```python
from build123d import *

# Parameters (mm, degrees)
BOSS_EXTRUDE1_DEPTH = 29.337
SKETCH1_R           = 5.842
BOSS_EXTRUDE2_DEPTH = 1.27
BOSS_EXTRUDE3_DEPTH = 12.7


with BuildPart() as part:
    # Sketch 1 → Boss-Extrude1 (new, symmetric)
    with BuildSketch(Plane.XY):
        Polygon((7.3025, 0), (3.65125, 6.324150511), (-3.65125, 6.324150511), (-7.3025, 0), (-3.65125, -6.324150511), (3.65125, -6.324150511), align=None)
    extrude(amount=BOSS_EXTRUDE1_DEPTH, both=True)

    # Sketch1 → Boss-Extrude2 (add)
    with BuildSketch(Plane(origin=(0, 0, -29.337), x_dir=(-1, 0, 0), z_dir=(0, 0, -1))):
        with Locations(Location((0, 0, 0), (0, 0, 180))):
            Circle(SKETCH1_R)
    extrude(amount=BOSS_EXTRUDE2_DEPTH)

    # Sketch2 → Boss-Extrude3 (add)
    with BuildSketch(Plane(origin=(0, 0, -30.607), x_dir=(-1, 0, 0), z_dir=(0, 0, -1))):
        Polygon((3.729553625, -6.278290851), (7.301936182, 0.090742758), (3.572382557, 6.369033609), (-3.729553625, 6.278290851), (-7.301936182, -0.090742758), (-3.572382557, -6.369033609), align=None)
    extrude(amount=BOSS_EXTRUDE3_DEPTH)


solid = part.part
```
Input: part model. Units: mm. Frame: model coordinates. Give positions to 0.01 mm unless a question says otherwise; leave off trailing zeros. Order: outer loops, then holes, each group sorted by start corner. A loop starts at its lowest first (then second) coordinate and runs counter-clockwise, first axis right, second up. Notation, with made-up numbers: M 0.25,-23 L 41.25,-23 A14 cw 41.25,-8 Z; hole C 15,-37 d2. An arc over 180 degrees is marked long. One line per question, with ' | ' between items.
1) Contact query for flat-ended pins moving along their axis: P1, Ø6, axis at x = -2, z = 17, coming from the -Y side; P2, Ø2, axis at x = -3.5, z = -1, coming from the +Y side; P3, Ø1, axis at x = -4.5, z = -6, coming from the +Y side. Output: stop coordinate, or through.
Filled in:
P1: stops at y = -6.32 | P2: stops at y = 6.32 | P3: stops at y = 5.72
2) Draft query along Z for faces 1 (the face through (0, 0, -43.307)), 2 (the face through (6, 0, -29.337)), 3 (the face through (0, 0, 29.337)), 4 (the face through (-5.46, 3.19, -36.87)). Return one class per face: pulls with the +Z half, pulls with the -Z half, needs draft (parallel to the pull), parting line crosses it, or undercut.
Filled in:
face 1: pulls with the -Z half | face 2: undercut | face 3: pulls with the +Z half | face 4: needs draft
3) Section A-A on y = -2.25. Output: boundary loops of the cut face in (x, z), and give its area (3 significant figures).
Filled in:
outline: M -6,-29.34 L -5.39,-29.34 L -5.39,-30.61 L -5.99,-30.61 L -5.99,-43.31 L 6.02,-43.31 L 6.02,-30.61 L 5.39,-30.61 L 5.39,-29.34 L 6,-29.34 L 6,29.34 L -6,29.34 Z | area: 871 mm2
4) Ray query, L1, parallel to Z at x = -4.25, y = 4.75; L2, parallel to Y at x = -1, z = -16; L3, parallel to Y at x = -5.25, z = 11. Return the intervals inside material, ascending.
Filled in:
L1: z = -43.31 to -30.61, -29.34 to 29.34 | L2: y = -6.32 to 6.32 | L3: y = -3.56 to 3.56
5) Section B-B on z = -32. Output: boundary loops of the cut face in (x, y), and give its area (3 significant figures).
Filled in:
outline: M -7.3,0.09 L -3.73,-6.28 L 3.57,-6.37 L 7.3,-0.09 L 3.73,6.28 L -3.57,6.37 Z | area: 139 mm2
6) Section C-C on y = 5. Output: boundary loops of the cut face in (x, z).
Filled in:
outline: M -4.42,-29.34 L -3.02,-29.34 L -3.02,-30.61 L -4.39,-30.61 L -4.39,-43.31 L 4.45,-43.31 L 4.45,-30.61 L 3.02,-30.61 L 3.02,-29.34 L 4.42,-29.34 L 4.42,29.34 L -4.42,29.34 Z
